The figure shows three views and two pictorial views of one solid part (mm, origin at its lowest corner). Answer the questions. A direction names the side the tool comes from. Coordinates: 2 decimals unless noted, no trailing zeros. Write each loop counter-clockwise with the first axis right and the second up, starting at its lowest first coordinate (ties: lowest second). Pieces come first, ordered by that corner, then holes. Notation, with made-up numbers: M 40.5,84.5 L 91.5,84.5 A17 ccw 91.5,113.5 Z; hole C 9,60.5 d11. An arc over 180 degrees is marked long. Answer as CSV lines item,"result".
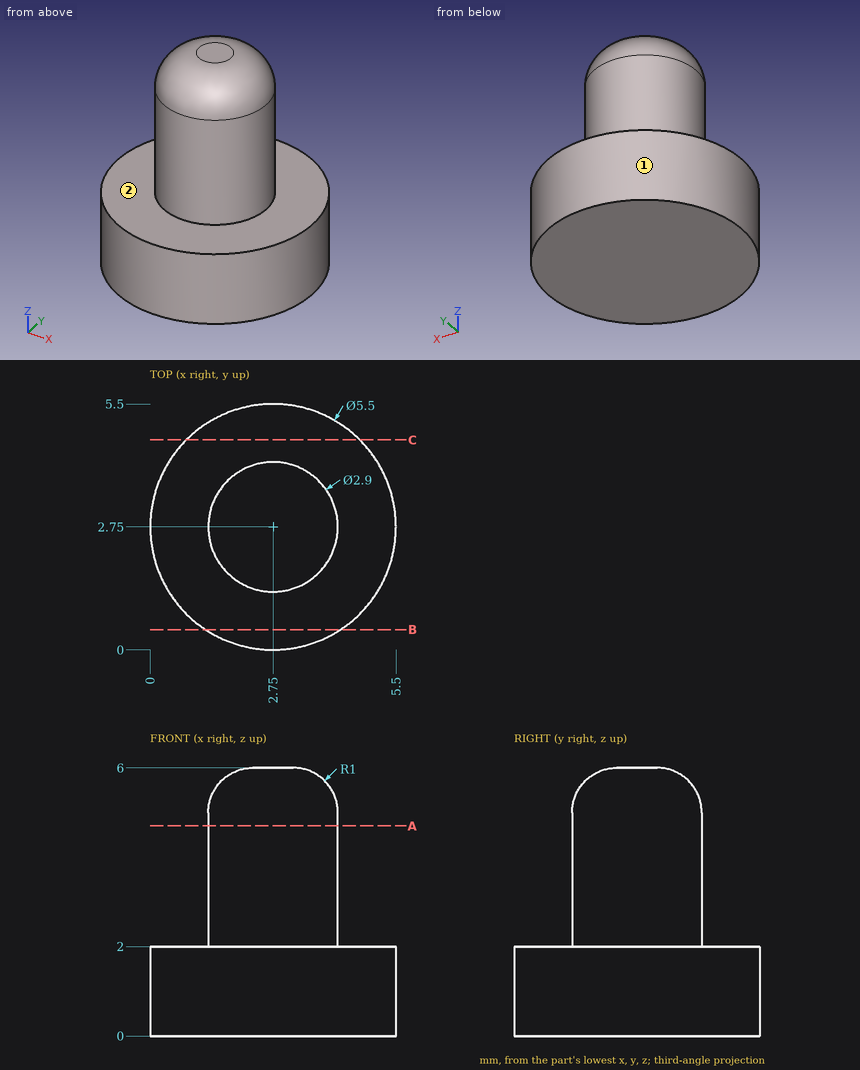
Q1. Straight lines are drawn through the part: line 1 (Z direction, x = 1.05, y = 4.35); line 2 (X direction, y = 2.15, z = 4); line 3 (Y direction, x = 2.95, z = 3.45). For each, find the intervals that lie inside material, in ascending order.
Output:
line 1,"0 to 2"
line 2,"1.43 to 4.07"
line 3,"1.31 to 4.19"
Q2. Find section A-A (z = 4.7). Give the vertices of the cut face in (x, y), and give its area (3 significant figures).
Output:
outline,"C 2.75,2.75 d2.9"
area,"6.61 mm2"
Q3. Find section C-C (y = 4.7). Give the vertices of the cut face in (x, z), and give its area (3 significant figures).
Output:
outline,"M 0.81,0 L 4.69,0 L 4.69,2 L 0.81,2 Z"
area,"7.76 mm2"
Q4. For the marked faces 1 and 2, determine the directions among +Z, -Z, +X, -X, +Y, -Y from which every point of the face is accessible in a straight line to the end or side of a thin tool.
Output:
face 1,"+Z, -Z"
face 2,"+Z"
Q5. Flat-ended cylindrical pins translate along their axes: pin 1 Ø1 at (y, z) = (2, 4) entering from +X; pin 2 Ø1 at (y, z) = (3.5, 2) entering from -X; pin 3 Ø3 at (x, z) = (4.5, 1) entering from -Y; pin 4 Ø3 at (x, y) = (2.5, 4) entering from +Z. Find the tip coordinate at first contact, or state that the pin passes through.
Output:
pin 1,"x = 4.18"
pin 2,"x = 0.01"
pin 3,"y = 0.01"
pin 4,"z = 6"
Q6. Find section B-B (y = 0.45). Give the vertices of the cut face in (x, z).
Output:
outline,"M 1.24,0 L 4.26,0 L 4.26,2 L 1.24,2 Z"
